Check sheet for the modelled part. Datum: model origin and axes. Units: mm. Face numbers are marked on the shaded views. Round coordinates to 2 decimals unless told otherwise and drop trailing zeros. Order: outer loops, then holes, each group sorted by start corner. A loop starts at its lowest first (then second) coordinate and runs counter-clockwise, first axis right, second up.
```python
from build123d import *

# Parameters (mm, degrees)
F0_W     = 60.325
F0_H     = 64.897
F1_DEPTH = 1.5875
F3_DEPTH = 3.175
F5_DEPTH = 3.175
F7_D     = 2.7051
F8_SIZE  = 2.54


with BuildPart() as f1:
    # F0 (on Top) → F1 (new body)
    with BuildSketch(Plane.XY):
        with Locations((30.1625, 32.4485)):
            Rectangle(F0_W, F0_H)
    extrude(amount=F1_DEPTH)

    # F2 (on face) → F3 (join)
    with BuildSketch(Plane(origin=(0, 0, 0), x_dir=(1, 0, 0), z_dir=(0, 0, -1))):
        Polygon((58.7375, -63.3095), (58.7375, -51.2445), (46.6725, -63.3095), align=None)
        Polygon((58.7375, -1.5875), (46.6725, -1.5875), (58.7375, -13.6525), align=None)
    extrude(amount=F3_DEPTH)

    # F4 (on face) → F5 (join)
    with BuildSketch(Plane(origin=(0, 0, 0), x_dir=(1, 0, 0), z_dir=(0, 0, -1))):
        Polygon((13.6525, -1.5875), (1.5875, -1.5875), (1.5875, -13.6525), align=None)
        Polygon((1.5875, -51.2445), (1.5875, -63.3095), (13.6525, -63.3095), align=None)
    extrude(amount=F5_DEPTH)

    # F7 (through all)
    with Locations(Plane.XY.offset(1.5875)):
        with Locations((54.7243, 59.2963), (54.7243, 5.6007), (5.6007, 5.6007), (5.6007, 59.2963)):
            Hole(F7_D / 2)

    # F8
    f8_edges = [f1.edges().sort_by_distance(p)[0] for p in [
        (46.6725, 1.5875, -1.5875),
        (58.7375, 13.6525, -1.5875),
        (58.7375, 51.2445, -1.5875),
        (46.6725, 63.3095, -1.5875),
        (13.6525, 1.5875, -1.5875),
        (1.5875, 13.6525, -1.5875),
        (1.5875, 51.2445, -1.5875),
        (13.6525, 63.3095, -1.5875),
    ]]
    chamfer(f8_edges, length=F8_SIZE)


solid = f1.part
```
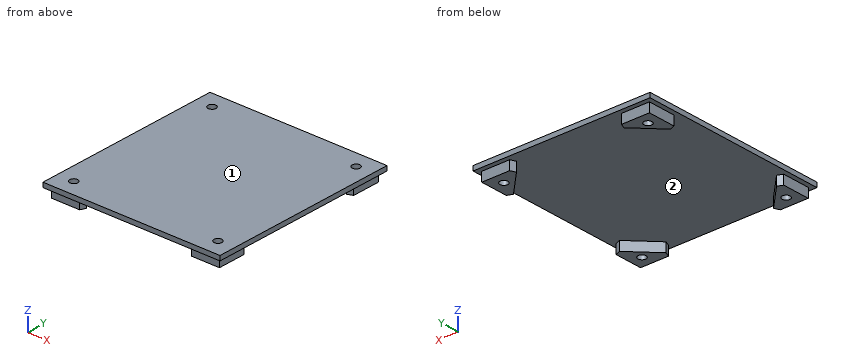
Item 1: Sectioned sample at D-D (x = 52.5). Record the cut outline in (y, z) (1 decimal).
Answer:
outline: (0, 0) - (1.6, 0) - (1.6, -3.2) - (7.4, -3.2) - (7.4, 0) - (57.5, 0) - (57.5, -3.2) - (63.3, -3.2) - (63.3, 0) - (64.9, 0) - (64.9, 1.6) - (0, 1.6) - close
Item 2: Sectioned sample at B-B (y = 22.5). Record the cut outline in (x, z) (1 decimal).
Answer:
outline: (0, 0) - (60.3, 0) - (60.3, 1.6) - (0, 1.6) - close
Item 3: Go/stop test with flat-tipped pins: P1, Ø1.5, axis at x = 16, z = -1, coming from the -Y side; P2, Ø10, axis at x = 20, y = 9, coming from the -Z side; P3, Ø1, axis at y = 8.5, z = -1.5, coming from the -X side; P4, Ø1, axis at x = 7, z = -2.5, coming from the -Y side. Record where each tip stops, or that it passes through.
Answer:
P1: passes through
P2: stops at z = 0
P3: stops at x = 1.59
P4: stops at y = 1.59
Item 4: Sectioned sample at C-C (x = 23.5). Record the cut outline in (y, z), and give its area (3 significant figures).
Answer:
outline: (0, 0) - (64.9, 0) - (64.9, 1.59) - (0, 1.59) - close
area: 103 mm2
Item 5: Sectioned sample at A-A (z = -1.5). Record the cut outline in (x, y), and give its area (3 significant figures).
Answer:
outline: (1.59, 1.59) - (11.11, 1.59) - (11.86, 3.38) - (3.38, 11.86) - (1.59, 11.11) - close; (1.59, 53.78) - (3.38, 53.04) - (11.86, 61.51) - (11.11, 63.31) - (1.59, 63.31) - close; (48.47, 3.38) - (49.21, 1.59) - (58.74, 1.59) - (58.74, 11.11) - (56.94, 11.86) - close; (48.47, 61.51) - (56.94, 53.04) - (58.74, 53.78) - (58.74, 63.31) - (49.21, 63.31) - close; hole circle Ø2.71 at (5.6, 5.6); hole circle Ø2.71 at (5.6, 59.3); hole circle Ø2.71 at (54.72, 5.6); hole circle Ø2.71 at (54.72, 59.3)
area: 250 mm2
Item 6: Release check for a two-part mould opening along Y. For the marked faces 1 and 2 record: released by +Y, released by -Y, zero draft, split by the parting line, or undercut.
Answer:
face 1: zero draft
face 2: undercut
Item 7: Scan lines: line 1 along Z through (x, y) = (27, 33.5); line 2 along X through (y, z) = (57.5, -0.75); line 3 along X through (y, z) = (6, 1.1) (3 decimals). Record each from-to range of solid material in increasing order.
Answer:
line 1: z = 0 to 1.59
line 2: x = 1.59 to 7.84, 52.48 to 58.74
line 3: x = 0 to 4.308, 6.893 to 53.432, 56.017 to 60.325
